Input: part model. Units: mm. Frame: model coordinates. Face numbers are marked on the shaded views. A direction names the side the tool comes from. Give positions to 0.01 mm unless a question says otherwise; leave off trailing zeros. Loops run counter-clockwise (first coordinate to the right, second up) from the corner with the lowest first, then second, coordinate; pieces in that order, holes last. Notation, with made-up numbers: (40.25, -3.5) - (49.25, -3.5) arc R30 ccw to (49.25, 22.5) - close; hole circle Ø1 at (-4, -31). An arc over 180 degrees is marked (long way). One line per item, written item: value.
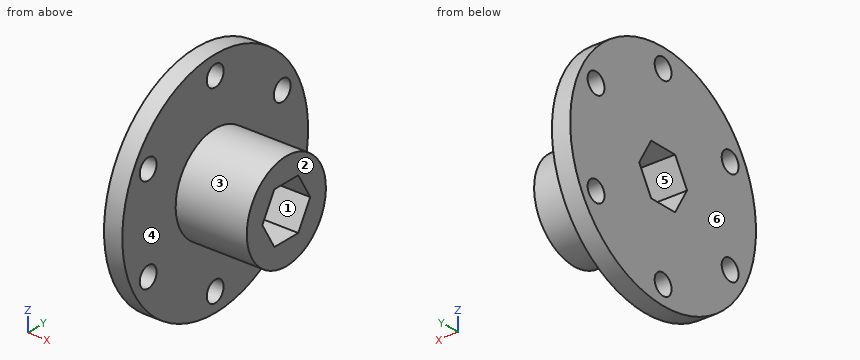
from build123d import *

# Parameters (mm, degrees)
SKETCH1_W           = 4.572
SKETCH1_H           = 28.575
SKETCH2_R           = 12.1666
BOSS_EXTRUDE1_DEPTH = 17.78
CUT_EXTRUDE1_DEPTH  = 47.180874331
HOLE1_D             = 5.1816
HOLE1_DEPTH         = 22.352


with BuildPart() as part:
    # Sketch1 → Revolve1 (revolve)
    with BuildSketch(Plane.XY, mode=Mode.PRIVATE) as revolve1_sk:
        with Locations((-15.321066246, 14.2875)):
            Rectangle(SKETCH1_W, SKETCH1_H)
    revolve(revolve1_sk.sketch.rotate(Axis((-17.607066246, 0, 0), (1, 0, 0)), 270), axis=Axis((-17.607066246, 0, 0), (1, 0, 0)))

    # Sketch2 → Boss-Extrude1 (add)
    with BuildSketch(Plane(origin=(-13.035066246, 0, 0), x_dir=(0, 0, -1), z_dir=(1, 0, 0))):
        Circle(SKETCH2_R)
    extrude(amount=BOSS_EXTRUDE1_DEPTH)

    # Sketch3 → Cut-Extrude1 (cut, through all)
    with BuildSketch(Plane.ZY.offset(17.607066246)):
        Polygon((0, -7.361697812), (6.3754, -3.680858906), (6.3754, 3.680818906), (0, 7.361657812), (-6.3754, 3.680818906), (-6.3754, -3.680858906), align=None)
    extrude(amount=-CUT_EXTRUDE1_DEPTH, mode=Mode.SUBTRACT)

    # Hole1
    with Locations(Plane.ZY.offset(17.607066246)):
        with Locations((11.90625, -20.622229928), (-11.90625, -20.622229928), (-23.8125, 0), (-11.90625, 20.622229928), (11.90625, 20.622229928), (23.8125, 0)):
            Hole(HOLE1_D / 2, depth=HOLE1_DEPTH)


solid = part.part
Item 1: Draft query along Z for the marked faces 1, 2 and 3. Return one class per face: pulls with the +Z half, pulls with the -Z half, needs draft (parallel to the pull), parting line crosses it, or undercut.
Verdict:
face 1: undercut
face 2: needs draft
face 3: parting line crosses it
Item 2: Section B-B, the plane x = -11. Output: boundary loops of the cut face in (y, z).
Verdict:
outline: circle Ø24.33 at (0, 0); hole (-7.36, 0) - (-3.68, -6.38) - (3.68, -6.38) - (7.36, 0) - (3.68, 6.38) - (-3.68, 6.38) - close
Item 3: Section D-D, the plane y = -9. Output: boundary loops of the cut face in (x, z), and give its area (3 significant figures).
Verdict:
outline: (-17.61, -27.12) - (-13.04, -27.12) - (-13.04, -8.19) - (4.74, -8.19) - (4.74, 8.19) - (-13.04, 8.19) - (-13.04, 27.12) - (-17.61, 27.12) - close
area: 539 mm^2
Item 4: Pin query (flat end, axial travel): P1, Ø6, axis at x = -9.5, y = 1.5, coming from the +Z side; P2, Ø6, axis at y = 1.5, z = -1, coming from the +X side; P3, Ø2, axis at x = -12.5, z = -9, coming from the -Y side; P4, Ø8.5, axis at y = 20.62, z = -11.91, coming from the +X side. Return the tip coordinate at first contact, or that it passes through.
Verdict:
P1: stops at z = 12.17
P2: passes through
P3: stops at y = -27.39
P4: stops at x = -13.04
Item 5: Section C-C, the plane z = 22. Output: boundary loops of the cut face in (x, y).
Verdict:
outline: (-17.61, -18.24) - (-13.04, -18.24) - (-13.04, -1.85) - (-17.61, -1.85) - close; (-17.61, 1.85) - (-13.04, 1.85) - (-13.04, 18.24) - (-17.61, 18.24) - close
Item 6: Material intervals for L1, parallel to Y at x = 2.75, z = 0; L2, parallel to X at y = 17.5, z = 16; L3, parallel to Z at x = -2.5, y = -3, sorted ascending.
Verdict:
L1: y = -12.17 to -7.36, 7.36 to 12.17
L2: x = -17.61 to -13.04
L3: z = -11.79 to -6.38, 6.38 to 11.79
Item 7: Section A-A, the plane y = 0. Output: boundary loops of the cut face in (x, z) (3 decimals).
Verdict:
outline: (-17.607, -28.575) - (-13.035, -28.575) - (-13.035, -26.403) - (-17.607, -26.403) - close; (-17.607, -21.222) - (-13.035, -21.222) - (-13.035, -12.167) - (4.745, -12.167) - (4.745, -6.375) - (-17.607, -6.375) - close; (-17.607, 6.375) - (4.745, 6.375) - (4.745, 12.167) - (-13.035, 12.167) - (-13.035, 21.222) - (-17.607, 21.222) - close; (-17.607, 26.403) - (-13.035, 26.403) - (-13.035, 28.575) - (-17.607, 28.575) - close
Item 8: Access query for the marked faces 4, 5 and 6. Directions: +Z, -Z, +X, -X, +Y, -Y. A direction counts if a zero-diameter tool reaches every point of the face in a straight line with its end or side. Return the directions, or none.
Verdict:
face 4: +X
face 5: +X, -X
face 6: +Z, -Z, -X, +Y, -Y
